```python
from build123d import *

# Parameters (mm, degrees)
F0_W     = 119.706568
F0_H     = 101.024038
F1_DEPTH = 25.4
F2_R     = 20.348716
F3_DEPTH = 32.004
F5_DEPTH = 63.5


with BuildPart() as f1:
    # F0 (on Top) → F1 (new body)
    with BuildSketch(Plane.XY):
        Rectangle(F0_W, F0_H)
    extrude(amount=F1_DEPTH)

    # F2 (on face) → F3 (join)
    with BuildSketch(Plane.XY.offset(25.4)):
        Circle(F2_R)
    extrude(amount=F3_DEPTH)

    # F4 (on Front) → F5 (cut, symmetric)
    with BuildSketch(Plane.XZ):
        Polygon((24.732081, 57.519987), (-22.998786, 57.519987), (24.732081, 38.122512), align=None)
    extrude(amount=F5_DEPTH, both=True, mode=Mode.SUBTRACT)


solid = f1.part
```
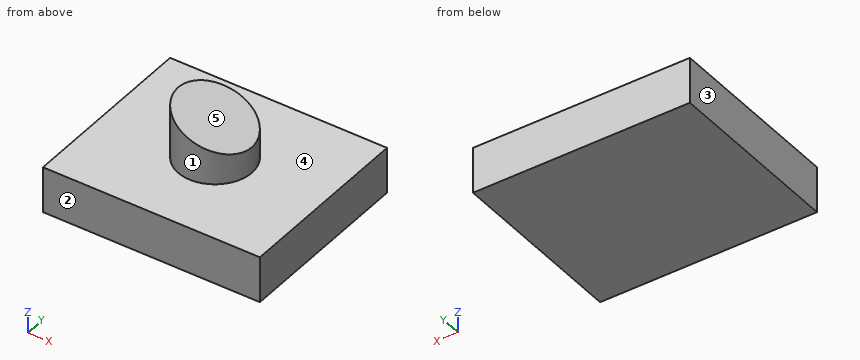
Check sheet for the modelled part. Datum: model origin and axes. Units: mm. Face numbers are marked on the shaded views. A direction names the side the tool comes from. Round coordinates to 2 decimals unless told otherwise and drop trailing zeros. Order: outer loops, then holes, each group sorted by start corner. A loop starts at its lowest first (then second) coordinate and runs counter-clockwise, first axis right, second up. Notation, with made-up numbers: (61, 28.25) -> (117, 28.25) arc R17 cw to (117, 45.25) -> close; hole circle Ø10 at (2, -11.5). An arc over 180 degrees is marked (long way). One line per item, written item: value. Start each with the question number.
Q1. Gauge pin test, flat ends, axial feed: pin 1 Ø1.5 at (x, y) = (-23, 11) entering from -Z; pin 2 Ø2 at (x, z) = (15.5, 30) entering from -Y; pin 3 Ø8 at (y, z) = (-10, 49.5) entering from -X; pin 4 Ø1.5 at (y, z) = (-7.5, 26.5) entering from +X. Record the tip position at first contact, or that the pin passes through.
Q2. Mould release check, pull along Y, two halves, no side actions. Record for the marked faces 1, 2 and 3: pulls with the +Y half, pulls with the -Y half, needs draft (parallel to the pull), parting line crosses it, or undercut.
Q3. Cross-section at D-D (x = -26). Record the boundary of the cut face in (y, z), and give its area (3 significant figures).
Q4. Set-up check for the marked faces 4 and 5: record each of +Z, -Z, +X, -X, +Y, -Y from which the full face is reachable in a straight line by a thin tool's end or side.
Q5. Cross-section at B-B (z = 33.5). Record the boundary of the cut face in (x, y), and give its area (3 significant figures).
Q6. Cross-section at A-A (y = 0). Record the boundary of the cut face in (x, z), and give its area (3 significant figures).
Q7. Thickness scan on line 1 (Z direction, x = 21, y = 34.5); line 2 (Y direction, x = 4, z = 37.5); line 3 (Z direction, x = -13, y = 12.5). Record the ranges inside material, lowest first.
Q8. Cross-section at C-C (x = 0). Record the boundary of the cut face in (y, z).
Completed:
1. pin 1: stops at z = 0
1. pin 2: stops at y = -14.28
1. pin 3: stops at x = -19.44
1. pin 4: stops at x = 19.2
2. face 1: parting line crosses it
2. face 2: pulls with the -Y half
2. face 3: needs draft
3. outline: (-50.51, 0) -> (50.51, 0) -> (50.51, 25.4) -> (-50.51, 25.4) -> close
3. area: 2,570 mm²
4. face 4: +Z
4. face 5: +Z, +X, +Y, -Y
5. outline: circle Ø40.7 at (0, 0)
5. area: 1,300 mm²
6. outline: (-59.85, 0) -> (59.85, 0) -> (59.85, 25.4) -> (20.35, 25.4) -> (20.35, 39.9) -> (-20.35, 56.44) -> (-20.35, 25.4) -> (-59.85, 25.4) -> close
6. area: 3,970 mm²
7. line 1: z = 0 to 25.4
7. line 2: y = -19.95 to 19.95
7. line 3: z = 0 to 53.46
8. outline: (-50.51, 0) -> (50.51, 0) -> (50.51, 25.4) -> (20.35, 25.4) -> (20.35, 48.17) -> (-20.35, 48.17) -> (-20.35, 25.4) -> (-50.51, 25.4) -> close
